Check sheet for the modelled part. Datum: model origin and axes. Units: mm. A direction names the side the tool comes from. Give positions to 0.01 mm unless a question says otherwise; leave off trailing zeros. Order: outer loops, then holes, each group sorted by start corner. A loop starts at its lowest first (then second) coordinate and runs counter-clockwise, first axis right, second up. Notation, with made-up numbers: (55.25, 3) -> (80.25, 3) arc R11 cw to (80.25, 19) -> close; hole circle Ø7 at (-32.5, 14). An arc over 180 degrees is marked (long way). Answer in a Markdown table with one row per item. Add a question column.
(1) Set-up check for faces 4 (the face through (-0.263, -8.183, 9.507)), 5 (the face through (0, -18, 4.1)), 6 (the face through (-4.9, -18, 5)), 7 (the face through (0, -18, 5.9)): record each of +Z, -Z, +X, -X, +Y, -Y from which the full face is reachable in a straight line by a thin tool's end or side.
(2) Cross-section at B-B (y = -16.75). Record the cut outline in (x, z).
(3) Cross-section at C-C (z = 5). Record the cut outline in (x, y), then the cut area to 3 significant figures.
(4) Release check for a two-part mould opening along Y. For faces 1 (the face through (-0.1, -17, 3.6)), 2 (the face through (0, -9, 10)), 3 (the face through (0.51, -8.76, 9.51)) record: released by +Y, released by -Y, zero draft, split by the parting line, or undercut.
(5) Thickness scan on L1, parallel to Y at x = -1.5, z = 9.45; L2, parallel to Z at x = -0.75, y = -8; L3, parallel to Y at x = -1.5, z = 9.2. Record the ranges inside material, lowest first. Write a range as [from, to].
(6) Go/stop test with flat-tipped pins: pin 1 (2.5 mm diameter, centred on x = -2, y = -14, fed in from +Z); pin 2 (6 mm diameter, centred on x = -2.5, z = 7, fed in from +Y); pin 3 (0.6 mm diameter, centred on x = 1, y = -18.5, fed in from +Z); pin 4 (1.5 mm diameter, centred on x = 3.5, z = 1.5, fed in from -Y). Record where each tip stops, or that it passes through.
(7) Cross-section at A-A (z = 3.5). Record the cut outline in (x, y).
```python
from build123d import *

# Parameters (mm, degrees)
BOSS_EXTRUDE1_DEPTH = 10
CUT_EXTRUDE1_DEPTH  = 1
FILLET1_R           = 2
SKETCH3_R           = 1.25
SKETCH3_R_2         = 0.7
CUT_EXTRUDE2_DEPTH  = 1
BOSS_EXTRUDE2_DEPTH = 2


with BuildPart() as part:
    # Sketch1 → Boss-Extrude1 (new body)
    with BuildSketch(Plane.XY):
        Polygon((-9.814954576, -17), (9.814954576, -17), (0, 0), align=None)
    extrude(amount=BOSS_EXTRUDE1_DEPTH)

    # Sketch2 → Cut-Extrude1 (cut)
    with BuildSketch(Plane.XY.offset(10)):
        with BuildLine():
            ThreePointArc((-4.55976672, -13.28190161), (-0.216174522, -15.38675653), (4.127417675, -13.28190161))
            ThreePointArc((4.127417675, -13.28190161), (4.053734797, -12.655479816), (3.427313004, -12.729162694))
            ThreePointArc((3.427313004, -12.729162694), (-0.216174522, -14.494754927), (-3.859662049, -12.729162694))
            ThreePointArc((-3.859662049, -12.729162694), (-4.486083842, -12.655479816), (-4.55976672, -13.28190161))
        make_face()
    extrude(amount=-CUT_EXTRUDE1_DEPTH, mode=Mode.SUBTRACT)

    # Fillet1
    # the kernel refuses this fillet: 2 mm, written as the material it takes off along each edge
    with BuildSketch(Plane(origin=(6.350852961, -15, 2), x_dir=(0, -1, 0), z_dir=(0, 0, -1))) as fillet1_piece_1_section:
        Polygon((0, 0), (FILLET1_R * 1.02, 0), (FILLET1_R * 1.02, -FILLET1_R * 1.76669182372), (-FILLET1_R * 0.51, -FILLET1_R * 0.88334591186), align=None)
    fillet1_piece_1 = extrude(amount=FILLET1_R * 1.02, mode=Mode.PRIVATE)
    fillet1_piece_1 = fillet1_piece_1 - Plane(origin=(6.350852961, -15, 2), x_dir=(-0.8660254037844387, 0.4999999999999999, 0), z_dir=(0, 0, -1)) * Sphere(FILLET1_R, mode=Mode.PRIVATE)
    add(fillet1_piece_1, mode=Mode.SUBTRACT)
    with BuildSketch(Plane(origin=(6.350852961, -15, 8), x_dir=(0, -1, 0), z_dir=(0, 0, 1))) as fillet1_piece_2_section:
        Polygon((0, 0), (FILLET1_R * 1.02, 0), (FILLET1_R * 1.02, FILLET1_R * 1.76669182372), (-FILLET1_R * 0.51, FILLET1_R * 0.88334591186), align=None)
    fillet1_piece_2 = extrude(amount=FILLET1_R * 1.02, mode=Mode.PRIVATE)
    fillet1_piece_2 = fillet1_piece_2 - Plane(origin=(6.350852961, -15, 8), x_dir=(-0.8660254037844387, 0.4999999999999999, 0), z_dir=(0, 0, 1)) * Sphere(FILLET1_R, mode=Mode.PRIVATE)
    add(fillet1_piece_2, mode=Mode.SUBTRACT)
    with BuildSketch(Plane(origin=(0, -4, 2), x_dir=(-0.8660254037844387, 0.5000000000000001, 0), z_dir=(0, 0, -1))) as fillet1_piece_3_section:
        Polygon((0, 0), (FILLET1_R * 1.02, 0), (FILLET1_R * 1.02, FILLET1_R * 1.76669182372), (-FILLET1_R * 0.51, FILLET1_R * 0.88334591186), align=None)
    fillet1_piece_3 = extrude(amount=FILLET1_R * 1.02, mode=Mode.PRIVATE)
    fillet1_piece_3 = fillet1_piece_3 - Plane(origin=(0, -4, 2), x_dir=(0, -1, 0), z_dir=(0, 0, -1)) * Sphere(FILLET1_R, mode=Mode.PRIVATE)
    add(fillet1_piece_3, mode=Mode.SUBTRACT)
    with BuildSketch(Plane(origin=(0, -4, 8), x_dir=(-0.8660254037844387, 0.5000000000000001, 0), z_dir=(0, 0, 1))) as fillet1_piece_4_section:
        Polygon((0, 0), (FILLET1_R * 1.02, 0), (FILLET1_R * 1.02, -FILLET1_R * 1.76669182372), (-FILLET1_R * 0.51, -FILLET1_R * 0.88334591186), align=None)
    fillet1_piece_4 = extrude(amount=FILLET1_R * 1.02, mode=Mode.PRIVATE)
    fillet1_piece_4 = fillet1_piece_4 - Plane(origin=(0, -4, 8), x_dir=(0, -1, 0), z_dir=(0, 0, 1)) * Sphere(FILLET1_R, mode=Mode.PRIVATE)
    add(fillet1_piece_4, mode=Mode.SUBTRACT)
    with BuildSketch(Plane(origin=(-6.350852961, -15, 8), x_dir=(0, -1, 0), z_dir=(0, 0, 1))) as fillet1_piece_5_section:
        Polygon((0, 0), (FILLET1_R * 1.02, 0), (FILLET1_R * 1.02, -FILLET1_R * 1.76669182372), (-FILLET1_R * 0.51, -FILLET1_R * 0.88334591186), align=None)
    fillet1_piece_5 = extrude(amount=FILLET1_R * 1.02, mode=Mode.PRIVATE)
    fillet1_piece_5 = fillet1_piece_5 - Plane(origin=(-6.350852961, -15, 8), x_dir=(0.8660254037844387, 0.4999999999999999, 0), z_dir=(0, 0, 1)) * Sphere(FILLET1_R, mode=Mode.PRIVATE)
    add(fillet1_piece_5, mode=Mode.SUBTRACT)
    with BuildSketch(Plane(origin=(-6.350852961, -15, 2), x_dir=(0, -1, 0), z_dir=(0, 0, -1))) as fillet1_piece_6_section:
        Polygon((0, 0), (FILLET1_R * 1.02, 0), (FILLET1_R * 1.02, FILLET1_R * 1.76669182372), (-FILLET1_R * 0.51, FILLET1_R * 0.88334591186), align=None)
    fillet1_piece_6 = extrude(amount=FILLET1_R * 1.02, mode=Mode.PRIVATE)
    fillet1_piece_6 = fillet1_piece_6 - Plane(origin=(-6.350852961, -15, 2), x_dir=(0.8660254037844387, 0.4999999999999999, 0), z_dir=(0, 0, -1)) * Sphere(FILLET1_R, mode=Mode.PRIVATE)
    add(fillet1_piece_6, mode=Mode.SUBTRACT)
    with BuildSketch(Plane(origin=(9.814954576, -17, 2), x_dir=(-1, 0, 0), z_dir=(0, 0, 1))) as fillet1_piece_7:
        with BuildLine():
            CenterArc((FILLET1_R * 1.73205080757, -FILLET1_R), FILLET1_R, 90, 120)
            Line((FILLET1_R * 0.866025403784, -FILLET1_R * 1.5), (0, 0))
            Line((0, 0), (FILLET1_R * 1.73205080757, 0))
        make_face()
    extrude(amount=6, mode=Mode.SUBTRACT)
    with BuildSketch(Plane(origin=(0, 0, 2), x_dir=(-0.5000000000000001, -0.8660254037844386, 0), z_dir=(0, 0, 1)), Plane(origin=(-9.814954576, -17, 2), x_dir=(1, 0, 0), z_dir=(0, 0, 1))) as fillet1_piece_8:
        with BuildLine():
            CenterArc((FILLET1_R * 1.73205080757, FILLET1_R), FILLET1_R, 150, 120)
            Line((FILLET1_R * 0.866025403784, FILLET1_R * 1.5), (0, 0))
            Line((0, 0), (FILLET1_R * 1.73205080757, 0))
        make_face()
    extrude(amount=6, mode=Mode.SUBTRACT)
    with BuildSketch(Plane(origin=(8.082903769, -14, 0), x_dir=(0, 0, 1), z_dir=(-0.5000000000000001, 0.8660254037844387, 0)), Plane(origin=(-1.732050808, -3, 0), x_dir=(0, 0, 1), z_dir=(-0.5000000000000001, -0.8660254037844387, 0)), Plane(origin=(-6.350852961, -17, 0), x_dir=(0, 0, 1), z_dir=(1, 0, 0))) as fillet1_piece_9:
        with BuildLine():
            CenterArc((FILLET1_R, -FILLET1_R), FILLET1_R, 90, 90)
            Line((0, -FILLET1_R), (0, 0))
            Line((0, 0), (FILLET1_R, 0))
        make_face()
    extrude(amount=12.701705922, mode=Mode.SUBTRACT)
    with BuildSketch(Plane(origin=(8.082903769, -14, 10), x_dir=(0, 0, -1), z_dir=(-0.5000000000000001, 0.8660254037844387, 0)), Plane(origin=(-6.350852961, -17, 10), x_dir=(0, 0, -1), z_dir=(1, 0, 0)), Plane(origin=(-1.732050808, -3, 10), x_dir=(0, 0, -1), z_dir=(-0.5000000000000001, -0.8660254037844387, 0))) as fillet1_piece_10:
        with BuildLine():
            CenterArc((FILLET1_R, FILLET1_R), FILLET1_R, 180, 90)
            Line((0, FILLET1_R), (0, 0))
            Line((0, 0), (FILLET1_R, 0))
        make_face()
    extrude(amount=12.701705922, mode=Mode.SUBTRACT)
    with BuildSketch(Plane(origin=(-0.216174522, -9.852596625, 10), x_dir=(-0.7848692976014117, -0.6196613475783904, 0), z_dir=(-0.6196613475783904, 0.7848692976014117, 0))) as fillet1_piece_11:
        with BuildLine():
            CenterArc((7.266210713, -2), FILLET1_R, 90, 60)
            Line((5.534159905, -1), (5.534159905, 0))
            Line((5.534159905, 0), (7.266210713, 0))
        make_face()
    revolve(axis=Axis((-0.216174522, -9.852596625, 10), (0, 0, 1)), revolution_arc=103.417183009, mode=Mode.SUBTRACT)
    with BuildSketch(Plane(origin=(3.77736534, -13.005532152, 10), x_dir=(0.7848692976014108, -0.6196613475783915, 0), z_dir=(-0.6196613475783915, -0.7848692976014108, 0))) as fillet1_piece_12:
        with BuildLine():
            CenterArc((2.178051609, -2), FILLET1_R, 90, 60)
            Line((0.446000801, -1), (0.446000801, 0))
            Line((0.446000801, 0), (2.178051609, 0))
        make_face()
    revolve(axis=Axis((3.77736534, -13.005532152, 10), (0, 0, 1)), revolution_arc=180, mode=Mode.SUBTRACT)
    with BuildSketch(Plane(origin=(-0.216174522, -9.852596625, 10), x_dir=(0.7848692976014113, -0.6196613475783908, 0), z_dir=(0.6196613475783908, 0.7848692976014113, 0))) as fillet1_piece_13:
        with BuildLine():
            CenterArc((2.910107495, 2), FILLET1_R, 270, 60)
            Line((4.642158302, 1), (4.642158302, 0))
            Line((4.642158302, 0), (2.910107495, 0))
        make_face()
    revolve(axis=Axis((-0.216174522, -9.852596625, 10), (0, 0, -1)), revolution_arc=103.417183009, mode=Mode.SUBTRACT)
    with BuildSketch(Plane(origin=(-4.209714384, -13.005532152, 10), x_dir=(0.7848692976014146, 0.6196613475783866, 0), z_dir=(0.6196613475783866, -0.7848692976014146, 0))) as fillet1_piece_14:
        with BuildLine():
            CenterArc((2.178051609, -2), FILLET1_R, 90, 60)
            Line((0.446000801, -1), (0.446000801, 0))
            Line((0.446000801, 0), (2.178051609, 0))
        make_face()
    revolve(axis=Axis((-4.209714384, -13.005532152, 10), (0, 0, 1)), revolution_arc=180, mode=Mode.SUBTRACT)

    # Sketch3 → Cut-Extrude2 (cut)
    # profile 1 of 2: a face of its own
    with BuildSketch(Plane.XY.offset(10)):
        with Locations((1.5, -8)):
            Circle(SKETCH3_R)
        with Locations((1.5, -8)):
            Circle(SKETCH3_R_2, mode=Mode.SUBTRACT)
    # profile 2 of 2: a face of its own
    with BuildSketch(Plane.XY.offset(10)):
        with Locations(Location((-1.5, -8, 0), (0, 0, 94.109031583))):
            Circle(SKETCH3_R)
        with Locations((-1.5, -8)):
            Circle(SKETCH3_R_2, mode=Mode.SUBTRACT)
    extrude(amount=-CUT_EXTRUDE2_DEPTH, mode=Mode.SUBTRACT)

    # Sketch4 → Boss-Extrude2 (add)
    with BuildSketch(Plane.XZ.offset(17)):
        with BuildLine():
            Line((-4, 5.9), (4, 5.9))
            ThreePointArc((4, 5.9), (4.9, 5), (4, 4.1))
            Line((4, 4.1), (-4, 4.1))
            ThreePointArc((-4, 4.1), (-4.9, 5), (-4, 5.9))
        make_face()
    extrude(amount=BOSS_EXTRUDE2_DEPTH)


solid = part.part
```
Answer below:
| question | item | result |
|---|---|---|
| 1 | face 4 | +Z |
| 1 | face 5 | -Z, +X, -X, -Y |
| 1 | face 6 | -X, -Y |
| 1 | face 7 | +Z, +X, -X, -Y |
| 2 | outline | (-7.32, 2) arc R0.97 ccw to (-6.35, 1.03) -> (6.35, 1.03) arc R0.97 ccw to (7.32, 2) -> (7.32, 8) arc R0.97 ccw to (6.35, 8.97) -> (-6.35, 8.97) arc R0.97 ccw to (-7.32, 8) -> close |
| 3 | outline | (-8.08, -14) arc R2 ccw to (-6.35, -17) -> (-4.9, -17) -> (-4.9, -19) -> (4.9, -19) -> (4.9, -17) -> (6.35, -17) arc R2 ccw to (8.08, -14) -> (1.73, -3) arc R2 ccw to (-1.73, -3) -> close |
| 3 | area | 178 mm² |
| 4 | face 1 | released by -Y |
| 4 | face 2 | zero draft |
| 4 | face 3 | undercut |
| 5 | L1 | y = [-16.38, -15.6], [-13.94, -9.25], [-8.7, -7.3], [-6.75, -3.84] |
| 5 | L2 | z = [0, 9] |
| 5 | L3 | y = [-16.6, -15.37], [-14.18, -9.25], [-8.7, -7.3], [-6.75, -3.4] |
| 6 | pin 1 | stops at z = 9.97 |
| 6 | pin 2 | stops at y = -2 |
| 6 | pin 3 | stops at z = 5.9 |
| 6 | pin 4 | stops at y = -17 |
| 7 | outline | (-8.08, -14) arc R2 ccw to (-6.35, -17) -> (6.35, -17) arc R2 ccw to (8.08, -14) -> (1.73, -3) arc R2 ccw to (-1.73, -3) -> close |
